Geometry check sheet. Reference: the model listing, model coordinates, mm. Face numbers are marked on the shaded views. A direction names the side the tool comes from. Coordinates: 2 decimals unless noted, no trailing zeros. Order: outer loops, then holes, each group sorted by start corner. A loop starts at its lowest first (then second) coordinate and runs counter-clockwise, first axis right, second up. Notation, with made-up numbers: (15.5, -20) - (26.5, -20) arc R29 ccw to (26.5, 10) - close; hole circle Ø10 at (55, 51). An arc over 180 degrees is marked (long way). Return JSON: item names as keys, results as strings. Group by question number.
Item 1: Section check A-A on x = -38.1. Enter the section's corners in (y, z).
Item 2: Section check B-B on z = 31.75. Enter the section's corners in (x, y) (1 decimal), then the cut area to 3 significant figures.
Item 3: Section check C-C on y = -53. Enter the section's corners in (x, z).
Item 4: Section check D-D on z = 8. Give the number of separate pieces and of enclosed holes in the cut face, then the cut area to 3 significant figures.
Item 5: Scan lines: probe 1 along Y at (x, z) = (-38.1, 16); probe 2 along Y at (x, z) = (-2, 21); probe 3 along X at (y, z) = (-50, 7). Record each from-to range of solid material in increasing order.
Item 6: Tool access check on the marked faces 1, 2 and 3. Record the directions out of +Z, -Z, +X, -X, +Y, -Y that give a thin tool (end or side, any length) a straight path to the whole face; none if there is none.
Item 7: Draft check along X on the marked faces 4, 5 and 6. Enter one of: pulls with the +X half, pulls with the -X half, needs draft (parallel to the pull), parting line crosses it, or undercut.
Item 8: Gauge pin test, flat ends, axial feed: pin 1 (5 mm diameter, centred on x = -11, z = 22, fed in from +Y); pin 2 (7.5 mm diameter, centred on x = 105.5, y = -2, fed in from +Z); pin 3 (6.5 mm diameter, centred on y = 48.5, z = 18.5, fed in from -X). Record the tip position at first contact, or that the pin passes through.
from build123d import *

# Parameters (mm, degrees)
F0_W           = 228.6
F0_H           = 127
F0_R           = 4.7625
F0_R_2         = 4.0005
F0_R_3         = 6.2865
F0_R_4         = 9.8425
F1_DEPTH       = 12.7
F2_R           = 11.1125
F2_R_2         = 6.2865
F3_DEPTH       = 25.4
F4_W           = 23.2800319791
F4_H           = 1.5875
F5_DEPTH       = 25.4
F6_W           = 12.7
F6_H           = 127
F7_DEPTH       = 12.7
F8_W           = 228.6
F8_H           = 12.7
F9_DEPTH       = 12.7
F10_R          = 3.175
F11_SIZE2      = 6.35
F11_SIZE       = 19.05
F12_R          = 3.175
F13_R          = 2.4765
F14_DEPTH      = 25.4
F14_DEPTH_BACK = 25.4


with BuildPart() as f1:
    # F0 (on Top) → F1 (new body)
    with BuildSketch(Plane.XY):
        Rectangle(F0_W, F0_H)
        with Locations((-101.6, -50.8)):
            Circle(F0_R, mode=Mode.SUBTRACT)
        with Locations((-17.9451, -17.9451)):
            Circle(F0_R_2, mode=Mode.SUBTRACT)
        with Locations((101.6, -50.8)):
            Circle(F0_R, mode=Mode.SUBTRACT)
        with Locations((17.9451, -17.9451)):
            Circle(F0_R_2, mode=Mode.SUBTRACT)
        with Locations((-38.1, 0)):
            Circle(F0_R_3, mode=Mode.SUBTRACT)
        with Locations((-17.9451, 17.9451)):
            Circle(F0_R_2, mode=Mode.SUBTRACT)
        with Locations((-101.6, 50.8)):
            Circle(F0_R, mode=Mode.SUBTRACT)
        Circle(F0_R_4, mode=Mode.SUBTRACT)
        with Locations((38.1, 0)):
            Circle(F0_R_3, mode=Mode.SUBTRACT)
        with Locations((17.9451, 17.9451)):
            Circle(F0_R_2, mode=Mode.SUBTRACT)
        with Locations((101.6, 50.8)):
            Circle(F0_R, mode=Mode.SUBTRACT)
    extrude(amount=F1_DEPTH)

    # F2 (on face) → F3 (join)
    with BuildSketch(Plane.XY.offset(12.7)):
        with Locations((-38.1, 0)):
            Circle(F2_R)
        with Locations((-38.1, 0)):
            Circle(F2_R_2, mode=Mode.SUBTRACT)
        with Locations((38.1, 0)):
            Circle(F2_R)
        with Locations((38.1, 0)):
            Circle(F2_R_2, mode=Mode.SUBTRACT)
    extrude(amount=F3_DEPTH)

    # F4 (on face) → F5 (cut, through all)
    with BuildSketch(Plane.XY.offset(38.1)):
        with Locations((53.7348873913, 0)):
            Rectangle(F4_W, F4_H)
        with BuildLine():
            Line((-37.5724840105, -0.79375), (-37.5724840105, 0.79375))
            Line((-37.5724840105, 0.79375), (-44.3361881937, 0.79375))
            ThreePointArc((-44.3361881937, 0.79375), (-44.3865, 0), (-44.3361881937, -0.79375))
            Line((-44.3361881937, -0.79375), (-37.5724840105, -0.79375))
        make_face()
        with BuildLine():
            ThreePointArc((-44.3361881937, -0.79375), (-44.3865, 0), (-44.3361881937, 0.79375))
            Line((-44.3361881937, 0.79375), (-49.1841155347, 0.79375))
            ThreePointArc((-49.1841155347, 0.79375), (-49.2125, 0), (-49.1841155347, -0.79375))
            Line((-49.1841155347, -0.79375), (-44.3361881937, -0.79375))
        make_face()
        with BuildLine():
            ThreePointArc((-49.1841155347, -0.79375), (-49.2125, 0), (-49.1841155347, 0.79375))
            Line((-49.1841155347, 0.79375), (-60.8525159895, 0.79375))
            Line((-60.8525159895, 0.79375), (-60.8525159895, -0.79375))
            Line((-60.8525159895, -0.79375), (-49.1841155347, -0.79375))
        make_face()
    extrude(amount=-F5_DEPTH, mode=Mode.SUBTRACT)

    # F6 (on face) → F7 (join)
    with BuildSketch(Plane.XY.offset(12.7)):
        with Locations((-82.55, 0)):
            Rectangle(F6_W, F6_H)
        with Locations((82.55, 0)):
            Rectangle(F6_W, F6_H)
    extrude(amount=F7_DEPTH)

    # F8 (on face) → F9 (join)
    with BuildSketch(Plane.XY.offset(12.7)):
        with Locations((0, -31.75)):
            Rectangle(F8_W, F8_H)
        with Locations((0, 31.75)):
            Rectangle(F8_W, F8_H)
    extrude(amount=F9_DEPTH)

    # F10
    f10_edges = [f1.edges().sort_by_distance(p)[0] for p in [
        (-114.3, -63.5, 6.35),
        (114.3, -63.5, 6.35),
        (-114.3, 63.5, 6.35),
        (114.3, 63.5, 6.35),
    ]]
    fillet(f10_edges, radius=F10_R)

    # F11
    f11_edges = [f1.edges().sort_by_distance(p)[0] for p in [
        (-114.3, 31.75, 25.4),
        (-114.3, -31.75, 25.4),
        (114.3, -31.75, 25.4),
        (114.3, 31.75, 25.4),
        (-82.55, -63.5, 25.4),
        (82.55, -63.5, 25.4),
        (82.55, 63.5, 25.4),
        (-82.55, 63.5, 25.4),
    ]]
    f11_side = f1.faces().sort_by_distance((78.81509, 50.8, 25.4))[0]
    chamfer(f11_edges, length=F11_SIZE, length2=F11_SIZE2, reference=f11_side)

    # F12
    f12_edges = [f1.edges().sort_by_distance(p)[0] for p in [
        (-114.3, -31.75, 19.05),
        (-114.3, 31.75, 19.05),
        (-95.25, 31.75, 25.4),
        (-95.25, -31.75, 25.4),
        (95.25, -31.75, 25.4),
        (114.3, -31.75, 19.05),
        (114.3, 31.75, 19.05),
        (95.25, 31.75, 25.4),
        (-82.55, -63.5, 19.05),
        (82.55, -63.5, 19.05),
        (82.55, -44.45, 25.4),
        (-82.55, -44.45, 25.4),
        (-82.55, 44.45, 25.4),
        (-82.55, 63.5, 19.05),
        (82.55, 44.45, 25.4),
        (82.55, 63.5, 19.05),
    ]]
    fillet(f12_edges, radius=F12_R)

    # F13 (on Front) → F14 (cut, two sides)
    with BuildSketch(Plane.XZ) as f14_sk:
        with Locations((-38.1, 31.75)):
            Circle(F13_R)
        with Locations((38.1, 31.75)):
            Circle(F13_R)
    extrude(amount=-F14_DEPTH, mode=Mode.SUBTRACT)
    extrude(f14_sk.sketch, amount=F14_DEPTH_BACK, mode=Mode.SUBTRACT)


solid = f1.part
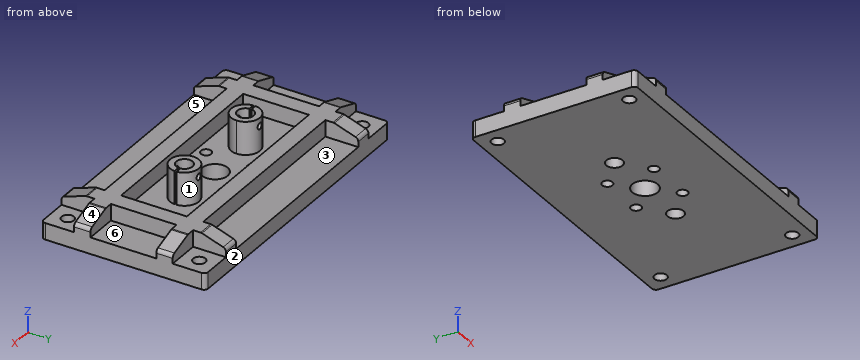
Computed:
{
 "1": {"outline": "(-63.5, 0) - (-6.29, 0) - (-6.29, 29.27) - (-11.11, 29.27) - (-11.11, 12.7) - (-25.4, 12.7) - (-25.4, 25.4) - (-38.1, 25.4) - (-38.1, 12.7) - (-63.5, 12.7) - close; (-11.11, 34.23) - (-6.29, 34.23) - (-6.29, 38.1) - (-11.11, 38.1) - close; (6.29, 0) - (63.5, 0) - (63.5, 12.7) - (38.1, 12.7) - (38.1, 25.4) - (25.4, 25.4) - (25.4, 12.7) - (11.11, 12.7) - (11.11, 29.27) - (6.29, 29.27) - close; (6.29, 34.23) - (11.11, 34.23) - (11.11, 38.1) - (6.29, 38.1) - close"},
 "2": {"outline": "(-49.2, -0.8) arc R11.1 ccw to (-40.6, -10.8) - (-40.6, -5.8) arc R6.3 cw to (-44.3, -0.8) - close; (-49.2, 0.8) - (-44.3, 0.8) arc R6.3 cw to (-40.6, 5.8) - (-40.6, 10.8) arc R11.1 ccw to start; (-35.6, -10.8) arc R11.1 ccw to (-35.6, 10.8) - (-35.6, 5.8) arc R6.3 cw to (-35.6, -5.8) - close; (35.6, -10.8) - (35.6, -5.8) arc R6.3 cw to (35.6, 5.8) - (35.6, 10.8) arc R11.1 ccw to start; (40.6, -10.8) arc R11.1 ccw to (49.2, -0.8) - (44.3, -0.8) arc R6.3 cw to (40.6, -5.8) - close; (40.6, 5.8) arc R6.3 cw to (44.3, 0.8) - (49.2, 0.8) arc R11.1 ccw to (40.6, 10.8) - close", "area": "415 mm²"},
 "3": {"outline": "(-114.3, 0) - (-105.82, 0) - (-105.82, 12.7) - (-114.3, 12.7) - close; (-97.38, 0) - (97.38, 0) - (97.38, 12.7) - (88.9, 12.7) - (88.9, 22.55) - (76.2, 22.55) - (76.2, 12.7) - (-76.2, 12.7) - (-76.2, 22.55) - (-88.9, 22.55) - (-88.9, 12.7) - (-97.38, 12.7) - close; (105.82, 0) - (114.3, 0) - (114.3, 12.7) - (105.82, 12.7) - close"},
 "4": {"separate pieces": "1", "enclosed holes": "11", "area": "28,000 mm²"},
 "5": {"probe 1": "y = -38.1 to -25.4, -11.11 to -6.29, 6.29 to 11.11, 25.4 to 38.1", "probe 2": "y = -38.1 to -25.4, 25.4 to 38.1", "probe 3": "x = -114.3 to -106.29, -96.91 to 96.91, 106.29 to 114.3"},
 "6": {"face 1": "+Z", "face 2": "+Z, -Z, +X, -X, +Y", "face 3": "+Z, +Y"},
 "7": {"face 4": "pulls with the +X half", "face 5": "undercut", "face 6": "needs draft"},
 "8": {"pin 1": "stops at y = 38.1", "pin 2": "stops at z = 12.7", "pin 3": "stops at x = -88.9"}
}
